Input: part model. Units: mm. Frame: model coordinates. Face numbers are marked on the shaded views. A direction names the side the tool comes from. Coordinates: 2 decimals unless noted, no trailing zeros. Order: outer loops, then holes, each group sorted by start corner. A loop starts at its lowest first (then second) coordinate and runs counter-clockwise, first axis right, second up.
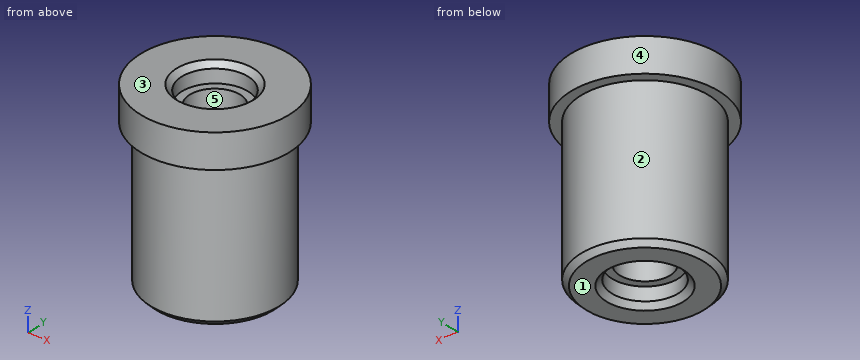
from build123d import *

# Parameters (mm, degrees)
SKETCH1_R           = 12.1
BOSS_EXTRUDE1_DEPTH = 17
SKETCH2_R           = 4.75
CUT_EXTRUDE1_DEPTH  = 39.063368217
SKETCH3_R           = 6.25
CUT_EXTRUDE2_DEPTH  = 3.5
SKETCH4_R           = 14
SKETCH4_R_2         = 12.1
SKETCH4_R_3         = 6.25
BOSS_EXTRUDE2_DEPTH = 6.35
CHAMFER1_SIZE       = 1


with BuildPart() as part:
    # Sketch1 → Boss-Extrude1 (new, symmetric)
    with BuildSketch(Plane.XY):
        Circle(SKETCH1_R)
    extrude(amount=BOSS_EXTRUDE1_DEPTH, both=True)

    # Sketch2 → Cut-Extrude1 (cut, through all)
    with BuildSketch(Plane.XY.offset(17)):
        Circle(SKETCH2_R)
    extrude(amount=-CUT_EXTRUDE1_DEPTH, mode=Mode.SUBTRACT)

    # Sketch3 → Cut-Extrude2 (cut)
    with BuildSketch(Plane.XY.offset(17)):
        Circle(SKETCH3_R)
    cut_extrude2 = extrude(amount=-CUT_EXTRUDE2_DEPTH, mode=Mode.SUBTRACT)

    # Mirror1: Cut-Extrude2 across plane
    add(cut_extrude2.mirror(Plane.XY), mode=Mode.SUBTRACT)

    # Sketch4 → Boss-Extrude2 (add)
    # profile 1 of 2: a face of its own
    with BuildSketch(Plane.XY.offset(17)):
        Circle(SKETCH4_R)
        Circle(SKETCH4_R_2, mode=Mode.SUBTRACT)
    # profile 2 of 2: a face of its own
    with BuildSketch(Plane.XY.offset(17)):
        Circle(SKETCH4_R_2)
        Circle(SKETCH4_R_3, mode=Mode.SUBTRACT)
    extrude(amount=-BOSS_EXTRUDE2_DEPTH)

    # Chamfer1
    chamfer1_edges = [part.edges().sort_by_distance(p)[0] for p in [
        (-6.25, 0, 17),
        (-6.25, 0, -17),
        (-12.1, 0, -17),
    ]]
    chamfer(chamfer1_edges, length=CHAMFER1_SIZE)


solid = part.part
Item 1: Access query for the marked faces 1 and 2. Directions: +Z, -Z, +X, -X, +Y, -Y. A direction counts if a zero-diameter tool reaches every point of the face in a straight line with its end or side. Return the directions, or none.
Response values:
face 1: -Z, +X, -X, +Y, -Y
face 2: -Z
Item 2: Cut plane C-C on z = 5. Return loops of the section in (x, y), then the cut area to 3 significant figures.
Response values:
outline: circle Ø24.2 at (0, 0); hole circle Ø9.5 at (0, 0)
area: 389 mm2
Item 3: Ray query, probe 1 along Y at (x, z) = (0, -14.2); probe 2 along Y at (x, z) = (0, 1); probe 3 along X at (y, z) = (3, -3.5). Return the intervals inside material, ascending.
Response values:
probe 1: y = -12.1 to -6.25, 6.25 to 12.1
probe 2: y = -12.1 to -4.75, 4.75 to 12.1
probe 3: x = -11.72 to -3.68, 3.68 to 11.72
Item 4: Cut plane A-A on x = 0. Return loops of the section in (y, z).
Response values:
outline: (-14, 10.65) - (-12.1, 10.65) - (-12.1, -16) - (-11.1, -17) - (-7.25, -17) - (-6.25, -16) - (-6.25, -13.5) - (-4.75, -13.5) - (-4.75, 13.5) - (-6.25, 13.5) - (-6.25, 16) - (-7.25, 17) - (-14, 17) - close; (4.75, -13.5) - (6.25, -13.5) - (6.25, -16) - (7.25, -17) - (11.1, -17) - (12.1, -16) - (12.1, 10.65) - (14, 10.65) - (14, 17) - (7.25, 17) - (6.25, 16) - (6.25, 13.5) - (4.75, 13.5) - close
Item 5: Draft query along Y for the marked faces 3, 4 and 5. Return one class per face: pulls with the +Y half, pulls with the -Y half, needs draft (parallel to the pull), parting line crosses it, or undercut.
Response values:
face 3: needs draft
face 4: parting line crosses it
face 5: undercut
Item 6: Pin query (flat end, axial travel): pin 1 Ø12 at (x, z) = (8, 2.5) entering from -Y; pin 2 Ø10 at (x, z) = (-5.5, 6) entering from -Y; pin 3 Ø4 at (x, y) = (3, 2) entering from +Z. Return the tip coordinate at first contact, or that it passes through.
Response values:
pin 1: stops at y = -11.93
pin 2: stops at y = -13.51
pin 3: stops at z = 13.5
